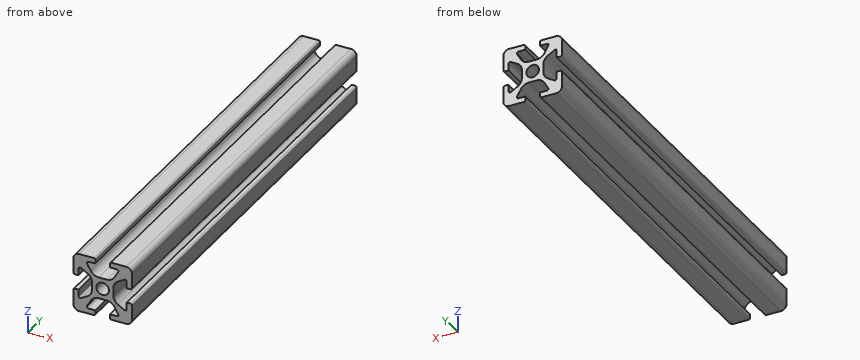
Solid Edge part; units mm, degrees
sketch "Sketch1" plane through (0, 0, 0) normal (0, -1, 0) x (1, 0, 0)
  line L0 (-10, -10) -> (10, -10)
  line L1 (10, -10) -> (10, 10)
  line L2 (10, 10) -> (-10, 10)
  line L3 (-10, 10) -> (-10, -10)
  dimension "D1" = 10
  dimension "D2" = 10
extrude "Protrusion1" add sketch "Sketch1" along normal mid plane 145
sketch "Sketch2" plane through (0, -72.5, 0) normal (0, -1, 0) x (1, 0, 0)
  line L0 (-2.5, 10) -> (-2.5, 8.2)
  line L1 (-2.5, 8.2) -> (-5.75, 8.2)
  line L2 (-5.75, 8.2) -> (-3.1231, 3.65)
  line L3 (-3.1231, 3.65) -> (3.1231, 3.65)
  line L4 (3.1231, 3.65) -> (5.75, 8.2)
  line L5 (5.75, 8.2) -> (2.5, 8.2)
  line L6 (2.5, 8.2) -> (2.5, 10)
  line L7 (2.5, 10) -> (-2.5, 10)
  dimension "D1" = 2.5
  dimension "D2" = 2.5
  dimension "D3" = 3.1231
extrude "Cutout1" cut sketch "Sketch2" against normal through all
fillet "Verrundung_1" radius 2 4 edges at (10, 0, 10) (-10, 0, 10) (10, 0, -10) (-10, 0, -10)
fillet "Verrundung_2" radius 3 2 edges at (-3.1231, 0, 3.65) (3.1231, 0, 3.65)
fillet "Verrundung_3" radius 0.5 4 edges at (-5.75, 0, 8.2) (5.75, 0, 8.2) (-2.5, 0, 10) (2.5, 0, 10)
hole "Bohrung_1" at (0, -72.5, 0) direction (0, 1, 0) diameter 4.3 end up to next
pattern_circular "Pattern1" count 4 over 360 about axis through (0, -72.5, 0) along (0, -1, 0) of "Cutout1"
fillet "Round1" radius 3 2 edges at (-3.65, 0, -3.1231) (-3.65, 0, 3.1231)
fillet "Round2" radius 0.5 4 edges at (-8.2, 0, -5.75) (-8.2, 0, 5.75) (-10, 0, -2.5) (-10, 0, 2.5)
fillet "Round3" radius 3 2 edges at (3.1231, 0, -3.65) (-3.1231, 0, -3.65)
fillet "Round4" radius 0.5 4 edges at (5.75, 0, -8.2) (-5.75, 0, -8.2) (2.5, 0, -10) (-2.5, 0, -10)
fillet "Round5" radius 3 2 edges at (3.65, 0, 3.1231) (3.65, 0, -3.1231)
fillet "Round6" radius 0.5 4 edges at (8.2, 0, 5.75) (8.2, 0, -5.75) (10, 0, 2.5) (10, 0, -2.5)
CAD build for the part. Positions are in the model's coordinates, mm. Give positions to 0.01 mm unless a question says otherwise; leave off trailing zeros. Loops run counter-clockwise (first coordinate to the right, second up) from the corner with the lowest first, then second, coordinate; pieces in that order, holes last. Notation, with made-up numbers: M 73.5,41.5 L 127.5,41.5 A25 cw 127.5,55.5 Z; hole C 77.5,89.25 d8. An arc over 180 degrees is marked long. Answer in a Markdown table with one row per item. Add a question column.
Item 1: Probe probe 1 along X at (y, z) = (3, 0); probe 2 along Z at (x, y) = (-7.75, -11.5). List the from-to ranges inside material, lowest first.
Item 2: Drop flat-ended pins along their axis: P1, Ø2, axis at y = -8, z = 0, coming from the -X side; P2, Ø3, axis at x = 0, y = -15, coming from the +Z side; P3, Ø1, axis at x = -9, y = -25.5, coming from the -Z side. Give the stop position or say it passes through.
Item 3: Band-saw the part on A-A on z = 0. Give the cut face in (x, y), then the cut area to 3 significant figures.
Reply:
| question | item | result |
|---|---|---|
| 1 | probe 1 | x = -3.65 to -2.15, 2.15 to 3.65 |
| 1 | probe 2 | z = -10 to -5.38, 5.38 to 10 |
| 2 | P1 | stops at x = -3.65 |
| 2 | P2 | stops at z = 3.65 |
| 2 | P3 | stops at z = -9.94 |
| 3 | outline | M -3.65,-72.5 L -2.15,-72.5 L -2.15,72.5 L -3.65,72.5 Z; M 2.15,-72.5 L 3.65,-72.5 L 3.65,72.5 L 2.15,72.5 Z |
| 3 | area | 435 mm^2 |
